The listing builds one solid part. Answer for the finished solid, in the listing's coordinates (mm). A direction names the side the tool comes from. Coordinates: 2 decimals unless noted, no trailing zeros. Write each loop counter-clockwise with the first axis right and the second up, starting at its lowest first coordinate (ties: lowest second). Pieces come first, ordered by that corner, then holes.
```python
from build123d import *

# Parameters (mm, degrees)
F0_R     = 25
F1_DEPTH = 50
F3_R     = 20
F4_R     = 20
F5_W     = 15
F5_H     = 15
F6_DEPTH = 40


with BuildPart() as f1:
    # F0 (on Front) → F1 (new body)
    with BuildSketch(Plane.XZ):
        Circle(F0_R)
    extrude(amount=F1_DEPTH)

    # F3
    f3_edges = [f1.edges().sort_by_distance(p)[0] for p in [
        (-25, -50, 0),
    ]]
    fillet(f3_edges, radius=F3_R)

    # F4
    f4_edges = [f1.edges().sort_by_distance(p)[0] for p in [
        (-25, 0, 0),
    ]]
    fillet(f4_edges, radius=F4_R)

    # F5 (on face) → F6 (join)
    with BuildSketch(Plane.XZ.offset(50)):
        Rectangle(F5_W, F5_H)
    extrude(amount=F6_DEPTH)


solid = f1.part
```
(1) Find the intervals of material crossed by probe 1 along X at (y, z) = (-84.5, 2); probe 2 along X at (y, z) = (-12.5, 15), in increasing order.
(2) Section A-A, the plane y = -65 is taken. Write down the section's boundary in (x, z), plus the area to 3 significant figures.
(3) Which of the six approach directions +Z, -Z, +X, -X, +Y, -Y give full straight-line access (tool end or side, diameter ignored) to faces 1 (the flat face through (0, -70, -7.5)), 2 (the flat face through (0, -70, 7.5)), 3 (the flat face through (7.5, -70, 0))?
(4) Each of these flat-tipped pins is pushed along its axis until it touches: pin 1 (1.5 mm diameter, centred on y = -23, z = 1.5, fed in from +X); pin 2 (5 mm diameter, centred on x = -19.5, z = 1.5, fed in from -Y); pin 3 (5 mm diameter, centred on x = 9, z = -14, fed in from +Y). Where does it stop, or does it pass through?
Solution:
1. probe 1: x = -7.5 to 7.5
1. probe 2: x = -18.14 to 18.14
2. outline: (-7.5, -7.5) - (7.5, -7.5) - (7.5, 7.5) - (-7.5, 7.5) - close
2. area: 225 mm2
3. face 1: -Z, +X, -X, -Y
3. face 2: +Z, +X, -X, -Y
3. face 3: +Z, -Z, +X, -Y
4. pin 1: stops at x = 24.99
4. pin 2: stops at y = -45.96
4. pin 3: stops at y = -2.21
